Autodesk Fusion 360 part; units mm, degrees
sketch "Sketch1" plane through (0, 0, 0) normal (0, 0, 1) x (1, 0, 0)
  line L0 (0, 0) -> (37.5, 0)
  line L1 (37.5, 0) -> (37.5, 30)
  line L2 (0, 0) -> (37.5, 0) construction
  line L3 (37.5, 30) -> (42.5, 30)
  line L4 (42.5, 30) -> (42.5, -40.5)
  line L5 (42.5, -40.5) -> (107.5, -40.5)
  line L6 (107.5, -40.5) -> (107.5, -157.5)
  line L7 (107.5, -157.5) -> (0, -157.5)
  line L8 (0, 0) -> (0, -157.5)
  dimension "d1" = 37.5
  dimension "d2" = 30
  dimension "d3" = 5
  dimension "d4" = 70.5
  dimension "d5" = 65
  dimension "d6" = 117
  dimension "d7" = 107.5
  dimension "d8" = 187.5
extrude "Extrude1" add sketch "Sketch1" along normal blind 5
equation "d1 = ( 75 / 2 ) * 1 mm"
equation "d5 = 20 mm + ( 15 * 3 ) * 1 mm"
equation "d6 = 67 mm + 20 mm + ( 10 * 3 ) * 1 mm"
equation "d7 = d1 + d3 + d5"
Check sheet for the modelled part. Datum: model origin and axes. Units: mm. A direction names the side the tool comes from. Round coordinates to 2 decimals unless told otherwise and drop trailing zeros. Write each loop counter-clockwise with the first axis right and the second up, starting at its lowest first coordinate (ties: lowest second). Pieces come first, ordered by that corner, then holes. Notation, with made-up numbers: (77.25, -26.75) - (117.25, -26.75) arc R24 cw to (117.25, -2.75) - close; hole circle Ø7 at (14, 42.5). An arc over 180 degrees is marked (long way). Return JSON: item names as keys, results as strings.
Q1. Cross-section at C-C (y = -13.5). Record the boundary of the cut face in (x, z), then the cut area to 4 significant figures.
Returned:
{"outline": "(0, 0) - (42.5, 0) - (42.5, 5) - (0, 5) - close", "area": "212.5 mm²"}
Q2. Cross-section at A-A (z = 2.5). Record the boundary of the cut face in (x, y).
Returned:
{"outline": "(0, -157.5) - (107.5, -157.5) - (107.5, -40.5) - (42.5, -40.5) - (42.5, 30) - (37.5, 30) - (37.5, 0) - (0, 0) - close"}
Q3. Scan lines: L1, parallel to Y at x = 82, z = 1.2; L2, parallel to Y at x = 11, z = 2; L3, parallel to X at y = 18.5, z = 0.75. Record each from-to range of solid material in increasing order. Write a range as from..to.
Returned:
{"L1": "y = -157.5..-40.5", "L2": "y = -157.5..0", "L3": "x = 37.5..42.5"}
Q4. Access from +Z, -Z, +X, -X, +Y, -Y to the whole of each face (thin tool, end or side, straight path). Record for faces 1 (the flat face through (18, 0, 2)), 2 (the flat face through (0, -78, 2)), 3 (the flat face through (75, -40.5, 2)).
Returned:
{"face 1": "+Z, -Z, -X, +Y", "face 2": "+Z, -Z, -X, +Y, -Y", "face 3": "+Z, -Z, +X, +Y"}
Q5. Cross-section at B-B (x = 74.5). Record the boundary of the cut face in (y, z).
Returned:
{"outline": "(-157.5, 0) - (-40.5, 0) - (-40.5, 5) - (-157.5, 5) - close"}
Q6. Depth check by flat-ended pin: P1, Ø2.5, axis at x = 88, z = 3, coming from the +Y side; P2, Ø2.5, axis at x = 11.5, z = 3, coming from the +Y side; P3, Ø2.5, axis at y = 2, z = 2.5, coming from the +X side. Enter the tip coordinate at first touch or a pass-through.
Returned:
{"P1": "stops at y = -40.5", "P2": "stops at y = 0", "P3": "stops at x = 42.5"}
